```python
from build123d import *

# Parameters (mm, degrees)
F0_R      = 50
F1_DEPTH  = 40
F2_R      = 45
F3_DEPTH  = 35
F4_W      = 10
F4_H      = 6
F5_DEPTH  = 50
F6_W      = 10
F6_H      = 6
F7_DEPTH  = 50
F8_W      = 10
F8_H      = 5.49967
F9_DEPTH  = 50
F10_W     = 10
F10_H     = 5.49967
F11_DEPTH = 50
F12_R     = 5.4
F13_DEPTH = 59
F14_R     = 5.4
F15_DEPTH = 55


with BuildPart() as f1:
    # F0 (on Top) → F1 (new body)
    with BuildSketch(Plane.XY):
        Circle(F0_R)
    extrude(amount=F1_DEPTH)

    # F2 (on face) → F3 (cut)
    with BuildSketch(Plane.XY.offset(40)):
        Circle(F2_R)
    extrude(amount=-F3_DEPTH, mode=Mode.SUBTRACT)

    # F4 (on Front) → F5 (cut)
    with BuildSketch(Plane.XZ):
        with Locations((0, 37)):
            Rectangle(F4_W, F4_H)
    extrude(amount=-F5_DEPTH, mode=Mode.SUBTRACT)

    # F6 (on Front) → F7 (cut)
    with BuildSketch(Plane.XZ):
        with Locations((0, 37)):
            Rectangle(F6_W, F6_H)
    extrude(amount=F7_DEPTH, mode=Mode.SUBTRACT)

    # F8 (on Right) → F9 (cut)
    with BuildSketch(Plane.YZ):
        with Locations((0, 37.250165)):
            Rectangle(F8_W, F8_H)
    extrude(amount=-F9_DEPTH, mode=Mode.SUBTRACT)

    # F10 (on Right) → F11 (cut)
    with BuildSketch(Plane.YZ):
        with Locations((0, 37.250165)):
            Rectangle(F10_W, F10_H)
    extrude(amount=F11_DEPTH, mode=Mode.SUBTRACT)

    # F12 (on Right) → F13 (cut)
    with BuildSketch(Plane.YZ):
        with Locations((-16.65, 14.419014)):
            Circle(F12_R)
        with Locations((16.65, 14.419014)):
            Circle(F12_R)
    extrude(amount=F13_DEPTH, mode=Mode.SUBTRACT)

    # F14 (on Right) → F15 (cut)
    with BuildSketch(Plane.YZ):
        with Locations((0, 15.636282)):
            Circle(F14_R)
    extrude(amount=-F15_DEPTH, mode=Mode.SUBTRACT)


solid = f1.part
```
Model file for the job. Use its own axes, mm. A direction names the side the tool comes from. Coordinates: 2 decimals unless noted, no trailing zeros. Order: outer loops, then holes, each group sorted by start corner. A loop starts at its lowest first (then second) coordinate and runs counter-clockwise, first axis right, second up. Notation, with made-up numbers: (-11.75, 2.25) -> (28.25, 2.25) arc R16 cw to (28.25, 33.25) -> close; hole circle Ø8 at (-21.5, -21.5). An arc over 180 degrees is marked (long way). Return JSON: item names as keys, results as strings.
Item 1: Pin check, flat tips, straight feed: P1, Ø4, axis at x = 47.5, z = 37.5, coming from the -Y side; P2, Ø4, axis at y = -48, z = 37.5, coming from the +X side; P3, Ø12, axis at x = 8.5, z = 27.5, coming from the -Y side. Stop position of each tip, or through.
Model answer:
{"P1": "stops at y = -20.73", "P2": "stops at x = 19.6", "P3": "stops at y = -49.94"}
Item 2: Mould opens along X. For faces 6 (the face through (46.187, -19.15, 19.72)), 7 (the face through (-47, 5, 37)), 8 (the face through (5, -47, 37)) say: pulls with the +X half, pulls with the -X half, needs draft (parallel to the pull), parting line crosses it, or undercut.
Model answer:
{"face 6": "parting line crosses it", "face 7": "needs draft", "face 8": "undercut"}
Item 3: Slice it at B-B (x = 0). Write the cut outline in (y, z), then the cut area to 3 significant figures.
Model answer:
{"outline": "(-50, 0) -> (50, 0) -> (50, 34) -> (45, 34) -> (45, 5) -> (-45, 5) -> (-45, 34) -> (-50, 34) -> close", "area": "790 mm²"}
Item 4: Slice it at D-D (z = 27.5). Write the cut outline in (x, y), then the cut area to 3 significant figures.
Model answer:
{"outline": "circle Ø100 at (0, 0); hole circle Ø90 at (0, 0)", "area": "1,490 mm²"}
Item 5: Slice it at A-A (y = 0). Write the cut outline in (x, z).
Model answer:
{"outline": "(-50, 0) -> (50, 0) -> (50, 34.5) -> (45, 34.5) -> (45, 5) -> (-45, 5) -> (-45, 10.24) -> (-50, 10.24) -> close; (-50, 21.04) -> (-45, 21.04) -> (-45, 34.5) -> (-50, 34.5) -> close"}
Item 6: 3-axis set-ups, long thin cutter, end or side, ignore diameter. For faces 1 (the face through (-33.17, 30.41, 22.74)), 2 (the face through (-47.3, 5, 13.6)), 3 (the face through (43.906, -22.045, 14.656)), 4 (the face through (47, -5, 37)), 5 (the face through (-5, 47, 37)): which of +Z, -Z, +X, -X, +Y, -Y reach the whole face in a straight line?
Model answer:
{"face 1": "+Z", "face 2": "-X", "face 3": "+X", "face 4": "+Z, +X, -X", "face 5": "+Z, +Y, -Y"}
Item 7: Wall check: line 1 along Z through (x, y) = (-8, -24.5); line 2 along Z through (x, y) = (45.5, -16.65); line 3 along X through (y, z) = (-22, 8). Give the ranges that are in metal, low to high. Write a range as from..to.
Model answer:
{"line 1": "z = 0..5", "line 2": "z = 0..9.02, 19.82..40", "line 3": "x = -44.9..-39.26, 39.26..44.9"}
Item 8: Slice it at C-C (y = -31). Write the cut outline in (x, z).
Model answer:
{"outline": "(-39.23, 0) -> (39.23, 0) -> (39.23, 40) -> (32.62, 40) -> (32.62, 5) -> (-32.62, 5) -> (-32.62, 40) -> (-39.23, 40) -> close"}
